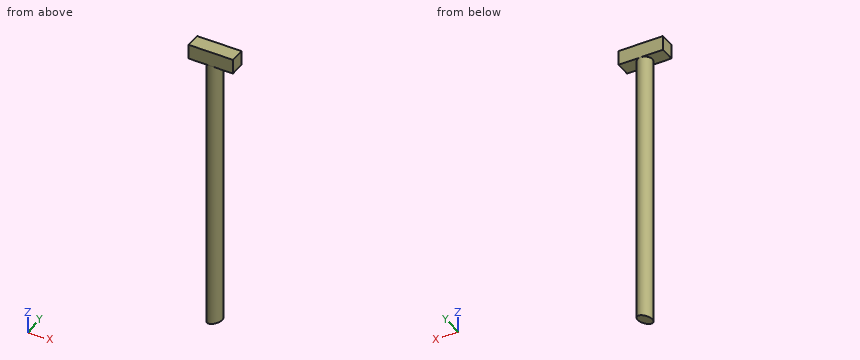
Autodesk Inventor part; units mm, degrees
ref_plane "Work Plane1" through (-15, 0, 200) normal (0, -1, 0) x (1, 0, 0)
ref_plane "YZ Plane" through (0, 0, 0) normal (1, 0, 0) x (0, 1, 0)
ref_plane "XZ Plane" through (0, 0, 0) normal (0, 1, 0) x (-1, 0, 0)
sketch "Sketch1" plane through (0, 0, 0) normal (0, 0, 1) x (1, 0, 0)
  circle A0 centre (0, 0) radius 5
  dimension "d0" = 10
extrude "Extrusion1" add sketch "Sketch1" along normal blind 200
sketch "Sketch2" plane through (0, 0, 0) normal (1, 0, 0) x (0, 1, 0)
  line L0 (-5, 0) -> (-5, 200)
  line L1 (5, 0) -> (5, 200)
  line L2 (5, 200) -> (-5, 200)
  line L3 (-5, 200) -> (5, 200)
  line L4 (5, 200) -> (5, 190)
  line L5 (5, 190) -> (-5, 190)
  line L6 (-5, 190) -> (-5, 200)
  point P0 (0, 0)
  dimension "d3" = 10
extrude "Extrusion2" add sketch "Sketch2" along normal mid plane 30
ref_plane "Work Plane1" through (-15, 0, 200) normal (0, -1, 0) x (1, 0, 0)
sketch "Sketch3" plane through (-15, 0, 200) normal (0, -1, 0) x (1, 0, 0)
  line L0 (0, 0) -> (30, 0)
  line L1 (30, -10) -> (30, 0)
  line L2 (15, -10) -> (30, -10)
  line L3 (0, -10) -> (15, -10)
  line L4 (0, 0) -> (0, -10)
  line L5 (15, -10) -> (15, -10)
  line L6 (15, -10) -> (15, -10)
  line L7 (10, -200) -> (20, -200)
  line L8 (20, -200) -> (20, -10)
  line L9 (10, -200) -> (20, -196.7508)
  line L10 (10, -200) -> (20, -200)
  line L11 (20, -196.7508) -> (20, -200)
  line L12 (10, -200) -> (20, -200)
  line L13 (10, -200) -> (10, -10)
  point P0 (15, -200)
  dimension "d10" = 18
extrude "Extrusion3" cut sketch "Sketch3" along normal through all both and the other way through all contours L9 L8 L7
properties part number "EE_Arm-Rod-Rev1"
Here's how the part is built. I have some questions about the finished solid (model axes, mm). Coordinates: 2 decimals unless noted, no trailing zeros. Order: outer loops, then holes, each group sorted by start corner. A loop starts at its lowest first (then second) coordinate and runs counter-clockwise, first axis right, second up. Notation, with made-up numbers: (56, -14) -> (103, -14) arc R11 cw to (103, 3) -> close; hole circle Ø8 at (55.25, 0). An arc over 180 degrees is marked (long way). Return JSON: item names as keys, results as strings.
1) If we section it at C-C on z = 161: List the corners of the cut face in (x, y) for me, plus the area to 3 significant figures.
Conclusion:
{"outline": "circle Ø10 at (0, 0)", "area": "78.5 mm²"}
2) If we section it at B-B on x = 8.75: List the corners of the cut face in (y, z) for me.
Conclusion:
{"outline": "(-5, 190) -> (5, 190) -> (5, 200) -> (-5, 200) -> close"}
3) If I drill on probe 1 along Z at (x, y) = (7.5, -2.5); probe 2 along X at (y, z) = (-0.5, 182); probe 3 along Z at (x, y) = (3, -1.25), over which ranges is the centre line in solid material (lowest first)?
Conclusion:
{"probe 1": "z = 190 to 200", "probe 2": "x = -4.97 to 4.97", "probe 3": "z = 2.6 to 200"}
4) If we section it at A-A on y = 0: List the corners of the cut face in (x, z) for me.
Conclusion:
{"outline": "(-15, 190) -> (-5, 190) -> (-5, 0) -> (5, 3.25) -> (5, 190) -> (15, 190) -> (15, 200) -> (-15, 200) -> close"}
5) I'm going to push flat-ended pins straight in: P1, Ø8, axis at x = 6, z = 142, coming from the -Y side; P2, Ø4, axis at x = 2.5, z = 66, coming from the +Y side; P3, Ø4, axis at y = 2.5, z = 148, coming from the -X side. Where does each tip first touch, or does it pass through?
Conclusion:
{"P1": "stops at y = -4.58", "P2": "stops at y = 4.97", "P3": "stops at x = -4.97"}
